Read the model definition and answer for the solid it produces. Units are mm, in the model's axes. Face numbers are marked on the shaded views. A direction names the side the tool comes from. Give positions to 0.01 mm unless a question says otherwise; leave off trailing zeros. Order: outer loops, then holes, each group sorted by start corner. A loop starts at its lowest first (then second) coordinate and runs counter-clockwise, first axis right, second up. Notation, with made-up numbers: (13, -39.5) - (69, -39.5) arc R11 ccw to (69, -19.5) - close; hole circle Ø6 at (-24.75, 20). An arc over 180 degrees is marked (long way). Answer as CSV lines item,"result". Start each with the question number.
from build123d import *

# Parameters (mm, degrees)
EXTRUDE_2_DEPTH     = 25
SKETCH_3_3_W        = 37.5
SKETCH_3_3_H        = 6
EXTRUDE_3_DEPTH     = 3
SKETCH_4_R          = 1.5
CUT_EXTRUDE_2_DEPTH = 4


with BuildPart() as part:
    # Sketch 3 → Extrude 2 (new body)
    with BuildSketch(Plane.XY):
        Polygon((101.7, 13), (101.7, 10), (37.5, 0), (0, 0), (-41.3, 10), (-41.3, 13), (0, 3), (37.5, 3), align=None)
    extrude(amount=EXTRUDE_2_DEPTH)

    # Sketch 3_3 → Extrude 3 (add)
    with BuildSketch(Plane.XY):
        with Locations((18.75, 6)):
            Rectangle(SKETCH_3_3_W, SKETCH_3_3_H)
    extrude(amount=EXTRUDE_3_DEPTH)

    # Sketch 4 → Cut-Extrude 2 (cut)
    with BuildSketch(Plane(origin=(0, 0, 0), x_dir=(-1, 0, 0), z_dir=(0, 0, -1))):
        with Locations((-3, 6)):
            Circle(SKETCH_4_R)
        with Locations((-34.5, 6)):
            Circle(SKETCH_4_R)
    extrude(amount=-CUT_EXTRUDE_2_DEPTH, mode=Mode.SUBTRACT)


solid = part.part
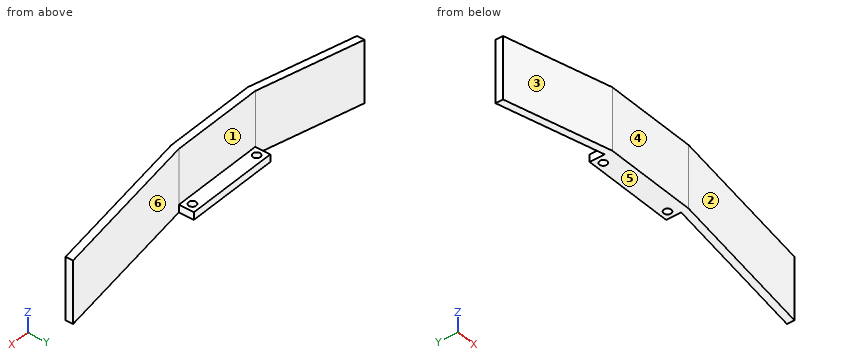
(1) Section C-C, the plane z = 1.75 is taken. Write down the section's boundary in (x, y), and give its area (3 significant figures).
(2) Straight lines are drawn through the part: line 1 (Z direction, x = 19, y = 6); line 2 (Y direction, x = 3, z = 1.2). For each, find the intervals that lie inside material, in ascending order. Write a range as [from, to].
(3) Section B-B, the plane x = 34.5 is taken. Write down the section's boundary in (y, z), and give its area (3 significant figures).
(4) Section A-A, the plane y = 6 is taken. Write down the section's boundary in (x, z), and give its area (3 significant figures).
(5) Flat-ended cylindrical pins translate along their axes: pin 1 Ø10 at (x, z) = (36.5, 8) entering from -Y; pin 2 Ø2 at (x, z) = (67.5, 19.5) entering from -Y; pin 3 Ø12 at (x, z) = (-3.5, 8.5) entering from +Y; pin 4 Ø12 at (x, z) = (-17.5, 13) entering from -Y. Find the tip coordinate at first contact, or state that the pin passes through.
(6) Section D-D, the plane z = 9.75 is taken. Write down the section's boundary in (x, y), and give its area (3 significant figures).
(7) Which of the six approach directions +Z, -Z, +X, -X, +Y, -Y give full straight-line access (tool end or side, diameter ignored) to the marked faces 5 and 6?
(8) Determine the mould class of the marked faces 1, 2, 3 and 4 for opening direction X: released by +X, released by -X, zero draft, split by the parting line, or undercut.
Checks:
1,outline,"(-41.3, 10) - (0, 0) - (37.5, 0) - (101.7, 10) - (101.7, 13) - (37.5, 3) - (37.5, 9) - (0, 9) - (0, 3) - (-41.3, 13) - close; hole circle Ø3 at (3, 6); hole circle Ø3 at (34.5, 6)"
1,area,"640 mm²"
2,line 1,"z = [0, 3]"
2,line 2,"y = [0, 4.5], [7.5, 9]"
3,outline,"(0, 0) - (4.5, 0) - (4.5, 3) - (3, 3) - (3, 25) - (0, 25) - close; (7.5, 0) - (9, 0) - (9, 3) - (7.5, 3) - close"
3,area,"84.0 mm²"
4,outline,"(-24.78, 0) - (-12.39, 0) - (-12.39, 25) - (-24.78, 25) - close; (0, 0) - (1.5, 0) - (1.5, 3) - (0, 3) - close; (4.5, 0) - (33, 0) - (33, 3) - (4.5, 3) - close; (36, 0) - (37.5, 0) - (37.5, 3) - (36, 3) - close; (56.76, 0) - (76.02, 0) - (76.02, 25) - (56.76, 25) - close"
4,area,"886 mm²"
5,pin 1,"stops at y = 0"
5,pin 2,"stops at y = 4.52"
5,pin 3,"stops at y = 5.3"
5,pin 4,"stops at y = 2.78"
6,outline,"(-41.3, 10) - (0, 0) - (37.5, 0) - (101.7, 10) - (101.7, 13) - (37.5, 3) - (0, 3) - (-41.3, 13) - close"
6,area,"429 mm²"
7,face 5,"-Z, +X, -X, +Y, -Y"
7,face 6,"+Z, -Z, +Y"
8,face 1,"undercut"
8,face 2,"released by +X"
8,face 3,"released by -X"
8,face 4,"zero draft"
